Geometry check sheet. Reference: the model listing, model coordinates, mm. A direction names the side the tool comes from. Give positions to 0.01 mm unless a question says otherwise; leave off trailing zeros. Loops run counter-clockwise (first coordinate to the right, second up) from the corner with the lowest first, then second, coordinate; pieces in that order, holes last. Notation, with made-up numbers: (-35.5, 20) - (-13.5, 20) arc R20 ccw to (-13.5, 33) - close; hole circle Ø4 at (31, 80). An arc over 180 degrees is marked (long way). Use a Markdown table: item, result. Add a question column.
1. Depth check by flat-ended pin: P1, Ø1.5, axis at y = 0, z = 7, coming from the +X side; P2, Ø12.5, axis at x = -0.5, y = -2, coming from the +Z side; P3, Ø4, axis at y = 2, z = 8, coming from the +X side; P4, Ø4, axis at x = -15.5, y = 15.5, coming from the -Z side. Enter the tip coordinate at first touch or a pass-through.
2. Cross-section at C-C on x = 11.5. Enter the section's corners in (y, z).
3. Cross-section at A-A on x = -15.5. Enter the section's corners in (y, z) (3 decimals).
4. Cross-section at D-D on z = 6.75. Enter the section's corners in (x, y) (3 decimals).
5. Material ranges on L1, parallel to X at y = 15.5, z = 7.25 (3 decimals); L2, parallel to Y at x = 10.5, z = 9.5; L3, parallel to Y at x = -6, z = 9, recorded low to high.
6. Cross-section at B-B on y = 0. Enter the section's corners in (x, z) (3 decimals), and give its area (3 significant figures).
7. Set-up check for faces 1 (the flat face through (13, 10, 5)), 2 (the cylindrical face through (-14.137, -16.065, 6.451)), 3 (the cylindrical face through (13.5, 17.4, 1.5)): record each of +Z, -Z, +X, -X, +Y, -Y from which the full face is reachable in a straight line by a thin tool's end or side.
from build123d import *

# Parameters (mm, degrees)
SKETCH004_R     = 1.475
PAD003_DEPTH    = 10
SKETCH009_R     = 2.76
POCKET002_DEPTH = 3
SKETCH014_R     = 11.1
POCKET006_DEPTH = 7


with BuildPart() as part:
    # Sketch004 → Pad003 (new body)
    with BuildSketch(Plane.XY):
        with BuildLine():
            Line((-21, 21), (21, 21))
            Line((21, 21), (21, 10))
            Line((21, 10), (0, 10))
            ThreePointArc((0, 10), (-10, 0), (0, -10))
            Line((21, -10), (0, -10))
            Line((21, -21), (21, -10))
            Line((21, -21), (-21, -21))
            Line((-21, -21), (-21, 21))
        make_face()
        with Locations((-15.5, 15.5)):
            Circle(SKETCH004_R, mode=Mode.SUBTRACT)
        with Locations((15.5, 15.5)):
            Circle(SKETCH004_R, mode=Mode.SUBTRACT)
        with Locations((-15.5, -15.5)):
            Circle(SKETCH004_R, mode=Mode.SUBTRACT)
        with Locations((15.5, -15.5)):
            Circle(SKETCH004_R, mode=Mode.SUBTRACT)
        with Locations((-15.5, 0)):
            Circle(SKETCH004_R, mode=Mode.SUBTRACT)
        with Locations((0, 15.5)):
            Circle(SKETCH004_R, mode=Mode.SUBTRACT)
        with Locations((0, -15.5)):
            Circle(SKETCH004_R, mode=Mode.SUBTRACT)
    extrude(amount=PAD003_DEPTH)

    # Sketch009 → Pocket002 (cut)
    with BuildSketch(Plane.XY):
        with Locations((-15.5, 15.5)):
            Circle(SKETCH009_R)
        with Locations((15.5, 15.5)):
            Circle(SKETCH009_R)
        with Locations((-15.5, -15.5)):
            Circle(SKETCH009_R)
        with Locations((15.5, -15.5)):
            Circle(SKETCH009_R)
        with Locations((-15.5, 0)):
            Circle(SKETCH009_R)
        with Locations((0, 15.5)):
            Circle(SKETCH009_R)
        with Locations((0, -15.5)):
            Circle(SKETCH009_R)
    extrude(amount=POCKET002_DEPTH, mode=Mode.SUBTRACT)

    # Sketch014 (on Face5 of Pocket002) → Pocket006 (cut)
    with BuildSketch(Plane.XY.offset(10)):
        Circle(SKETCH014_R)
    extrude(amount=-POCKET006_DEPTH, mode=Mode.SUBTRACT)


solid = part.part
Values found:
| question | item | result |
|---|---|---|
| 1 | P1 | stops at x = -11.07 |
| 1 | P2 | passes through |
| 1 | P3 | stops at x = -10.35 |
| 1 | P4 | stops at z = 3 |
| 2 | outline | (-21, 0) - (-10, 0) - (-10, 10) - (-21, 10) - close; (10, 0) - (21, 0) - (21, 10) - (10, 10) - close |
| 3 | outline | (-21, 0) - (-18.26, 0) - (-18.26, 3) - (-16.975, 3) - (-16.975, 10) - (-21, 10) - close; (-14.025, 3) - (-12.74, 3) - (-12.74, 0) - (-2.76, 0) - (-2.76, 3) - (-1.475, 3) - (-1.475, 10) - (-14.025, 10) - close; (1.475, 3) - (2.76, 3) - (2.76, 0) - (12.74, 0) - (12.74, 3) - (14.025, 3) - (14.025, 10) - (1.475, 10) - close; (16.975, 3) - (18.26, 3) - (18.26, 0) - (21, 0) - (21, 10) - (16.975, 10) - close |
| 4 | outline | (-21, -21) - (21, -21) - (21, -10) - (4.818, -10) arc R11.1 cw (long way) to (4.818, 10) - (21, 10) - (21, 21) - (-21, 21) - close; hole circle Ø2.95 at (-15.5, -15.5); hole circle Ø2.95 at (-15.5, 0); hole circle Ø2.95 at (-15.5, 15.5); hole circle Ø2.95 at (0, -15.5); hole circle Ø2.95 at (0, 15.5); hole circle Ø2.95 at (15.5, -15.5); hole circle Ø2.95 at (15.5, 15.5) |
| 5 | L1 | x = -21 to -16.975, -14.025 to -1.475, 1.475 to 14.025, 16.975 to 21 |
| 5 | L2 | y = -21 to -10, 10 to 21 |
| 5 | L3 | y = -21 to -9.34, 9.34 to 21 |
| 6 | outline | (-21, 0) - (-18.26, 0) - (-18.26, 3) - (-16.975, 3) - (-16.975, 10) - (-21, 10) - close; (-14.025, 3) - (-12.74, 3) - (-12.74, 0) - (-10, 0) - (-10, 3) - (-11.1, 3) - (-11.1, 10) - (-14.025, 10) - close |
| 6 | area | 65.1 mm2 |
| 7 | face 1 | +Z, -Z, +X |
| 7 | face 2 | +Z, -Z |
| 7 | face 3 | -Z |
